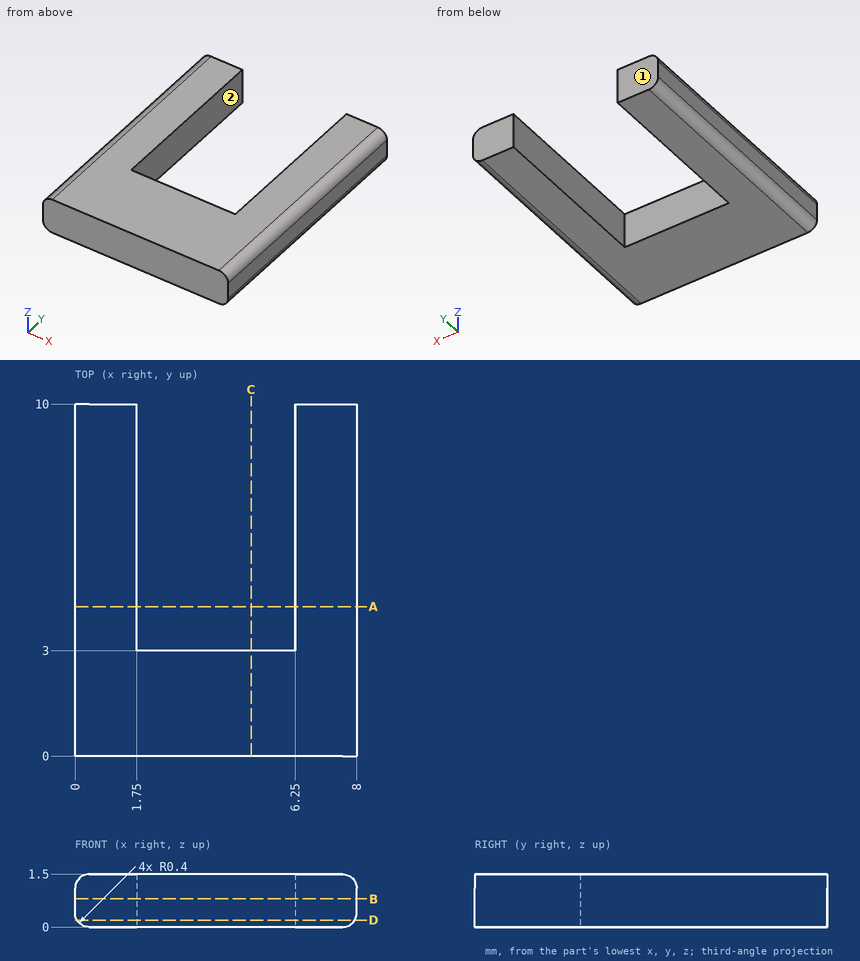
Can you work these out from the drawing? Everything is in mm from the part's minimum corner. A direction names the side the tool comes from. Coordinates: 2 decimals unless noted, no trailing zeros. Write each loop counter-clockwise with the first axis right and the second up, starting at its lowest first coordinate (ties: lowest second). Pieces come first, ordered by that corner, then holes. Notation, with made-up numbers: (-15.5, 59.5) - (-3.5, 59.5) arc R18 ccw to (-3.5, 86.5) - close; hole circle Ø3 at (-16.5, 29.5). An arc over 180 degrees is marked (long way). Use a Markdown table: item, result.
Q1. Which directions (+Z, -Z, +X, -X, +Y, -Y) give clear straight access to the entire face, cutting with the end or side of a thin tool? Please do the marked faces 1 and 2.
Geometry check:
| item | result |
|---|---|
| face 1 | +Z, -Z, +X, -X, +Y |
| face 2 | +Z, -Z, +Y |
Q2. Imagine slicing it at A-A (y = 4.25). List the corners of the cut face in (x, z) for me.
Geometry check:
| item | result |
|---|---|
| outline | (0, 0.4) arc R0.4 ccw to (0.4, 0) - (1.75, 0) - (1.75, 1.5) - (0.4, 1.5) arc R0.4 ccw to (0, 1.1) - close; (6.25, 0) - (7.6, 0) arc R0.4 ccw to (8, 0.4) - (8, 1.1) arc R0.4 ccw to (7.6, 1.5) - (6.25, 1.5) - close |
Q3. Please list where these lines run through material, in increasing order: L1, parallel to X at y = 5, z = 0.4; L2, parallel to Y at x = 4.5, z = 0.5; L3, parallel to X at y = 0.5, z = 0.35.
Geometry check:
| item | result |
|---|---|
| L1 | x = 0 to 1.75, 6.25 to 8 |
| L2 | y = 0 to 3 |
| L3 | x = 0 to 8 |
Q4. Imagine slicing it at B-B (z = 0.8). List the corners of the cut face in (x, y) for me, and give its area (3 significant figures).
Geometry check:
| item | result |
|---|---|
| outline | (0, 0) - (8, 0) - (8, 10) - (6.25, 10) - (6.25, 3) - (1.75, 3) - (1.75, 10) - (0, 10) - close |
| area | 48.5 mm2 |
Q5. Imagine slicing it at D-D (z = 0.2). List the corners of the cut face in (x, y) for me.
Geometry check:
| item | result |
|---|---|
| outline | (0.05, 0) - (7.95, 0) - (7.95, 10) - (6.25, 10) - (6.25, 3) - (1.75, 3) - (1.75, 10) - (0.05, 10) - close |
Q6. Imagine slicing it at C-C (x = 5). List the corners of the cut face in (y, z) for me.
Geometry check:
| item | result |
|---|---|
| outline | (0, 0) - (3, 0) - (3, 1.5) - (0, 1.5) - close |
